from build123d import *
from build123d.topology import SkipClean

# Parameters (mm, degrees)
SKETCH1_R                = 1.5
BOSS_EXTRUDE1_DEPTH      = 2.5
BOSS_EXTRUDE2_DEPTH      = 1.8
BOSS_EXTRUDE2_DEPTH_BACK = 2.5
SKETCH2_R                = 4.5
SKETCH2_R_2              = 1.5
SKETCH4_R                = 2.5
CUT_EXTRUDE1_DEPTH       = 2
BOSS_EXTRUDE3_START      = 0.75
SKETCH5_R                = 4.5
SKETCH5_R_2              = 2.5
BOSS_EXTRUDE3_DEPTH      = 0.75
SKETCH6_W                = 46.6
SKETCH6_H                = 25
BOSS_EXTRUDE4_DEPTH      = 2.5
CUT_EXTRUDE2_REACH       = 71.694


with BuildPart() as part:
    # Sketch1 → Boss-Extrude1 (new body)
    with BuildSketch(Plane(origin=(0, 0, 0), x_dir=(0, 0, -1), z_dir=(1, 0, 0))):
        with BuildLine():
            Line((0, 12.5), (42.5, 12.5))
            Line((42.5, 12.5), (42.5, -12.5))
            Line((42.5, -12.5), (0, -12.5))
            ThreePointArc((0, -12.5), (-12.5, 0), (0, 12.5))
        make_face()
        Circle(SKETCH1_R, mode=Mode.SUBTRACT)
    extrude(amount=BOSS_EXTRUDE1_DEPTH)

    # Sketch2 → Boss-Extrude2 (add, two sides: drawn at the far end of the back side and taken through both)
    with BuildSketch(Plane.ZY.offset(-BOSS_EXTRUDE2_DEPTH_BACK)):
        Circle(SKETCH2_R)
        Circle(SKETCH2_R_2, mode=Mode.SUBTRACT)
    extrude(amount=BOSS_EXTRUDE2_DEPTH + BOSS_EXTRUDE2_DEPTH_BACK)

    # Sketch4 → Cut-Extrude1 (cut)
    with BuildSketch(Plane(origin=(2.5, 0, 0), x_dir=(0, 0, -1), z_dir=(1, 0, 0))):
        Circle(SKETCH4_R)
    extrude(amount=-CUT_EXTRUDE1_DEPTH, mode=Mode.SUBTRACT)

    # Sketch5 → Boss-Extrude3 (add)
    with SkipClean():  # the faces are left unmerged after this step: merging them gives an invalid solid
        with BuildSketch(Plane(origin=(2.5, 0, 0), x_dir=(0, 0, -1), z_dir=(1, 0, 0)).offset(BOSS_EXTRUDE3_START)):
            with Locations(Location((0, 0, 0), (0, 0, 180))):
                Circle(SKETCH5_R)
            Circle(SKETCH5_R_2, mode=Mode.SUBTRACT)
        extrude(amount=-BOSS_EXTRUDE3_DEPTH)

    # Sketch6 → Boss-Extrude4 (add)
    with SkipClean():  # the faces are left unmerged after this step: merging them gives an invalid solid
        with BuildSketch(Plane(origin=(0, 0, -42.5), x_dir=(-1, 0, 0), z_dir=(0, 0, -1))):
            with Locations((20.8, 0)):
                Rectangle(SKETCH6_W, SKETCH6_H)
        extrude(amount=-BOSS_EXTRUDE4_DEPTH)
    add(part.part.scale(1), mode=Mode.REPLACE)  # the faces are merged on a copy

    # Sketch7 → Cut-Extrude2 (cut, up to next)
    with BuildSketch(Plane.XY.offset(-40), mode=Mode.PRIVATE) as cut_extrude2_sk1:
        with BuildLine():
            Line((-27.5, 12.5), (-36.5, 12.5))
            Line((-36.5, 12.5), (-36.5, 3))
            ThreePointArc((-36.5, 3), (-35.767766953, 1.232233047), (-34, 0.5))
            Line((-34, 0.5), (-28.16190379, 0.5))
            ThreePointArc((-28.16190379, 0.5), (-25.333476665, -0.376894374), (-23.497142274, -2.7))
            ThreePointArc((-23.497142274, -2.7), (-10.315341562, -4.242640687), (-16.5, 7.5))
            Line((-16.5, 7.5), (-22.5, 7.5))
            ThreePointArc((-22.5, 7.5), (-26.035533906, 8.964466094), (-27.5, 12.5))
        make_face()
    cut_extrude2_tool1 = extrude(cut_extrude2_sk1.sketch, amount=-CUT_EXTRUDE2_REACH, mode=Mode.PRIVATE) & part.part
    add(cut_extrude2_tool1.solids().sort_by_distance((-22.661838, 2.786009, -40))[0], mode=Mode.SUBTRACT)


solid = part.part
Design review of the part built by this model. Coordinates are the model's own, in mm. A direction names the side the tool comes from. Round coordinates to 2 decimals unless told otherwise and drop trailing zeros. Write each loop counter-clockwise with the first axis right and the second up, starting at its lowest first coordinate (ties: lowest second). Pieces come first, ordered by that corner, then holes.
Item 1: For faces 5 (the flat face through (0.5, -2, 0)), 6 (the flat face through (-1.8, -2, 0)), 7 (the cylindrical face through (-26, 8.93, -41.23)), 8 (the cylindrical face through (-0.89, 4.46, -0.59)), 9 (the cylindrical face through (-35.787, 1.252, -41.232)), list the 3-axis set-ups (+Z, -Z, +X, -X, +Y, -Y) from which the entire face can be reached by the end or side of a thin tool; tool diameter is ignored.
Item 2: For pin 1 Ø3 at (x, z) = (-31, -41.5) entering from +Y; pin 2 Ø2.5 at (y, z) = (-0.5, -0.5) entering from +X; pin 3 Ø12 at (y, z) = (-8.5, -6.5) entering from -X, all flat-tipped, find the tip position at first contact; note any pin that passes through.
Item 3: Consider section D-D on x = -21. Give the boundary of the cut face in (y, z).
Item 4: Consider section A-A on x = -15. Give the boundary of the cut face in (y, z).
Item 5: Draft analysis for pull direction Z (two halves, no side actions). For faces 1 (the cylindrical face through (-25.37, -0.35, -41.23)), 2 (the cylindrical face through (1.232, -0.275, 12.497)), 3 (the flat face through (-26, -3, -42.5)), 4 (the flat face through (0, 0, -14)), state which applies: released by +Z, released by -Z, zero draft, split by the parting line, or undercut.
Item 6: Wall thickness on L1, parallel to Z at x = -24, y = -8.75; L2, parallel to X at y = -6, z = -27; L3, parallel to X at y = 0, z = -40.9: over which ranges is each line inside the solid? List them lowest first.
Item 7: Consider section B-B on y = 6. Give the boundary of the cut face in (x, z).
Item 8: Consider section C-C on z = -16.5. Give the boundary of the cut face in (x, y), and give its area (3 significant figures).
Check values:
1. face 5: +X
1. face 6: +Z, -X, +Y, -Y
1. face 7: +Z, -Z
1. face 8: -X
1. face 9: +Z, -Z, +Y
2. pin 1: stops at y = 0.5
2. pin 2: stops at x = 0.5
2. pin 3: stops at x = 0
3. outline: (-12.5, -42.5) - (-6, -42.5) - (-6, -40) - (-12.5, -40) - close; (7.5, -42.5) - (12.5, -42.5) - (12.5, -40) - (7.5, -40) - close
4. outline: (-12.5, -42.5) - (-7.35, -42.5) - (-7.35, -40) - (-12.5, -40) - close; (7.35, -42.5) - (12.5, -42.5) - (12.5, -40) - (7.35, -40) - close
5. face 1: zero draft
5. face 2: released by +Z
5. face 3: released by -Z
5. face 4: undercut
6. L1: z = -42.5 to -40
6. L2: x = 0 to 2.5
6. L3: x = -44.1 to -25.98, -9 to 2.5
7. outline: (-44.1, -42.5) - (-36.5, -42.5) - (-36.5, -40) - (-44.1, -40) - close; (-12, -42.5) - (2.5, -42.5) - (2.5, 10.97) - (0, 10.97) - (0, -40) - (-12, -40) - close
8. outline: (0, -12.5) - (2.5, -12.5) - (2.5, 12.5) - (0, 12.5) - close
8. area: 62.5 mm2
